Read the model definition and answer for the solid it produces. Units are mm, in the model's axes. Give positions to 0.01 mm unless a question says otherwise; leave off trailing zeros. Order: outer loops, then holes, each group sorted by start corner. A loop starts at its lowest first (then second) coordinate and runs counter-clockwise, first axis right, second up.
Item 1: A cutting plane is placed at A-A (y = 56). Write down the section's boundary in (x, z), plus the area to 3 significant figures.
Item 2: A cutting plane is placed at B-B (z = 311.5). Write down the section's boundary in (x, y).
Item 3: Given pin 1 Ø4 at (y, z) = (-30, 385.5) entering from +X; pin 2 Ø6 at (y, z) = (-37.5, 231.5) entering from -X; pin 3 Ø9 at (x, y) = (0, 0) entering from +Z, each flat-ended and moving along its own axis, determine where each tip first touches the part or whether it passes through.
Item 4: Find the intervals of material crossed by line 1 along Z through (x, y) = (-9, -9); line 2 along Z through (x, y) = (32, -39.5); line 3 along Y through (x, z) = (0, 433), in increasing order.
Item 5: A cutting plane is placed at C-C (x = -33). State how many separate pieces and enclosed holes the cut face has, plus the area to 3 significant figures.
from build123d import *

# Parameters (mm, degrees)
EXTRUDEASSE_DEPTH      = 468
EXTRUDEASSE_DEPTH_BACK = 15
SKETCH1_R              = 65
SKETCH6_W              = 125.765742684
SKETCH6_H              = 20
CUT_EXTRUDE1_DEPTH     = 10


with BuildPart() as part:
    # Sketch1 → ExtrudeAsse (new, two sides: drawn at the far end of the back side and taken through both)
    with BuildSketch(Plane.XY.offset(-EXTRUDEASSE_DEPTH_BACK)):
        Circle(SKETCH1_R)
    extrude(amount=EXTRUDEASSE_DEPTH + EXTRUDEASSE_DEPTH_BACK)

    # Sketch3 → Cut-Revolve1 (revolve, cut)
    with BuildSketch(Plane(origin=(0, 0, 0), x_dir=(0, 0, -1), z_dir=(0.7071067811865414, -0.7071067811865537, 0)), mode=Mode.PRIVATE) as cut_revolve1_sk:
        Polygon((-227.7, -65), (-227.7, 10), (-232.7, 12.886751346), (-232.7, 0), (-232.7, -65), align=None)
    revolve(cut_revolve1_sk.sketch.rotate(Axis((0, 0, 232.7), (-0.7071067811865537, -0.7071067811865414, 0)), 90), axis=Axis((0, 0, 232.7), (-0.7071067811865537, -0.7071067811865414, 0)), mode=Mode.SUBTRACT)

    # Sketch3<3> → Cut-Revolve2 (revolve, cut)
    with BuildSketch(Plane(origin=(0, 0, 0), x_dir=(0, 0, -1), z_dir=(0.7071067811865414, -0.7071067811865537, 0)), mode=Mode.PRIVATE) as cut_revolve2_sk:
        Polygon((-340.5, 10), (-340.5, -65), (-335.5, -65), (-335.5, 10), (-340.5, 12.886751346), align=None)
    revolve(cut_revolve2_sk.sketch.rotate(Axis((7.071067812, 7.071067812, 340.5), (-0.7071067811865537, -0.7071067811865415, 0)), 90), axis=Axis((7.071067812, 7.071067812, 340.5), (-0.7071067811865537, -0.7071067811865415, 0)), mode=Mode.SUBTRACT)

    # Sketch4 → Cut-Revolve5 (revolve, cut)
    with BuildSketch(Plane(origin=(0, 0, 0), x_dir=(0, 0, -1), z_dir=(1, 0, 0)), mode=Mode.PRIVATE) as cut_revolve5_sk:
        Polygon((-468, 0), (-197.77110668, 0), (-194.884355334, 0), (-197.77110668, -5), (-468, -5), align=None)
    revolve(cut_revolve5_sk.sketch.rotate(Axis((0, 0, 0), (0, 0, 1)), 225), axis=Axis((0, 0, 0), (0, 0, 1)), mode=Mode.SUBTRACT)

    # Sketch5 → Cut-Revolve6 (revolve, cut)
    with BuildSketch(Plane(origin=(0, 0, 0), x_dir=(0, 0, -1), z_dir=(1, 0, 0)), mode=Mode.PRIVATE) as cut_revolve6_sk:
        Polygon((15, -5), (15, 0), (-162.113248654, 0), (-165, 0), (-162.113248654, -5), align=None)
    revolve(cut_revolve6_sk.sketch.rotate(Axis((0, 0, 0), (0, 0, 1)), 270), axis=Axis((0, 0, 0), (0, 0, 1)), mode=Mode.SUBTRACT)

    # Sketch3<5> → Cut-Revolve7 (revolve, cut)
    with BuildSketch(Plane(origin=(0, 0, 0), x_dir=(0, 0, -1), z_dir=(0.7071067811865414, -0.7071067811865537, 0)), mode=Mode.PRIVATE) as cut_revolve7_sk:
        Polygon((-124.9, 10), (-124.9, 12.886751346), (-119.9, 10), (-119.9, -65), (-124.9, -65), align=None)
    revolve(cut_revolve7_sk.sketch.rotate(Axis((-45.961940777, -45.961940777, 124.9), (0.7071067811865537, 0.7071067811865415, 0)), 270), axis=Axis((-45.961940777, -45.961940777, 124.9), (0.7071067811865537, 0.7071067811865415, 0)), mode=Mode.SUBTRACT)

    # Sketch6 → Cut-Extrude1 (cut)
    with BuildSketch(Plane(origin=(0, 0, 0), x_dir=(-1, 0, 0), z_dir=(0, 0, -1))):
        with Locations((-8.867505506, -35.961940777)):
            Rectangle(SKETCH6_W, SKETCH6_H)
    extrude(amount=CUT_EXTRUDE1_DEPTH, mode=Mode.SUBTRACT)


solid = part.part
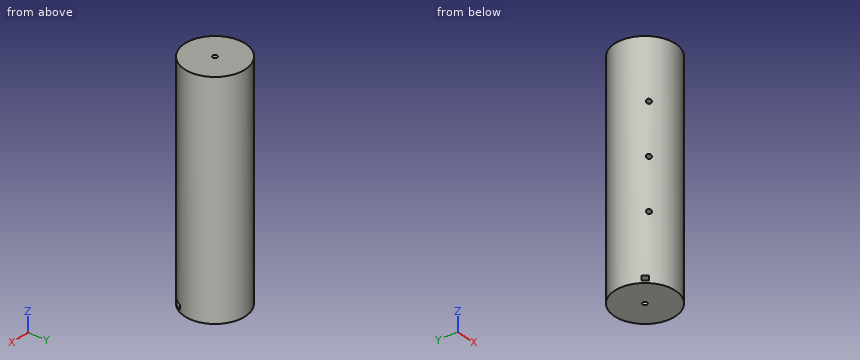
Response values:
1. outline: (-33, -15) - (33, -15) - (33, 468) - (-33, 468) - close
1. area: 31,900 mm2
2. outline: circle Ø130 at (0, 0); hole circle Ø10 at (0, 0)
3. pin 1: stops at x = 58.66
3. pin 2: stops at x = -55.09
3. pin 3: stops at z = 197.48
4. line 1: z = -15 to 119.9, 129.9 to 227.7, 237.7 to 335.5, 345.5 to 468
4. line 2: z = -15 to -10, 0 to 468
4. line 3: y = -65 to -5, 5 to 65
5. separate pieces: 1
5. enclosed holes: 4
5. area: 53,600 mm2
